Autodesk Inventor part; units mm, degrees
ref_plane "YZ Plane" through (0, 0, 0) normal (1, 0, 0) x (0, 1, 0)
ref_plane "XZ Plane" through (0, 0, 0) normal (0, 1, 0) x (-1, 0, 0)
ref_plane "XY Plane" through (0, 0, 0) normal (0, 0, 1) x (1, 0, 0)
sketch "Sketch1" plane through (0, 0, 0) normal (0, 0, 1) x (1, 0, 0)
  line L0 (0, 0) -> (3.75, 0)
  line L1 (3.75, 0) -> (3.75, -5)
  line L2 (3.75, -5) -> (11.25, -5)
  line L3 (11.25, -5) -> (11.25, 0)
  line L4 (11.25, 0) -> (21.731, 0)
  line L5 (21.731, 0) -> (21.731, 50)
  line L6 (21.731, 50) -> (11.25, 50)
  line L7 (11.25, 50) -> (11.25, 55)
  line L8 (11.25, 55) -> (3.75, 55)
  line L9 (3.75, 55) -> (3.75, 50)
  line L10 (3.75, 50) -> (0, 50)
  line L11 (0, 50) -> (0, 0)
  line L12 (21.731, 35) -> (15, 35)
  line L13 (15, 35) -> (15, 15)
  line L14 (15, 15) -> (21.731, 15)
  line L15 (21.731, 15) -> (21.731, 35)
  circle A0 centre (7.5, 35) radius 1.6
  circle A1 centre (7.5, 15) radius 1.6
  line L16 (7.5, 15) -> (7.5, 35)
  point P0 (21.731, 25)
  point P1 (21.731, 25)
  point P2 (7.5, -5)
  point P3 (7.5, 25)
  point P4 (0, 25)
  dimension "d0" = 50
  dimension "d1" = 3.75
  dimension "d2" = 5
  dimension "d3" = 7.5
  dimension "d4" = 10.481
  dimension "d5" = 6.731
  dimension "d6" = 20
  dimension "d7" = 3.75
  dimension "d10" = 3.2
  dimension "d11" = 20
extrude "Extrusion1" add sketch "Sketch1" along normal blind 6.731 contours L11 L10 L9 L8 L7 L6 L5 L12 L13 L14 L4 L3 L2 L1 L0
equation "\"d4\" = d7 + THICKB"
equation "\"d5\" = THICKB"
equation "\"d7\" = d1"
equation "\"d8\" = THICKB"
equation "\"THICKA\" = 3.175"
equation "\"THICKB\" = 6.731"
equation "\"THICKC\" = 12.7"
equation "\"BALLDIA\" = 12"
equation "\"MAGDIA\" = 9.5"
equation "\"THICKPLY\" = 5"
properties part number "Frame_Lower_Vertical_Plate_A"
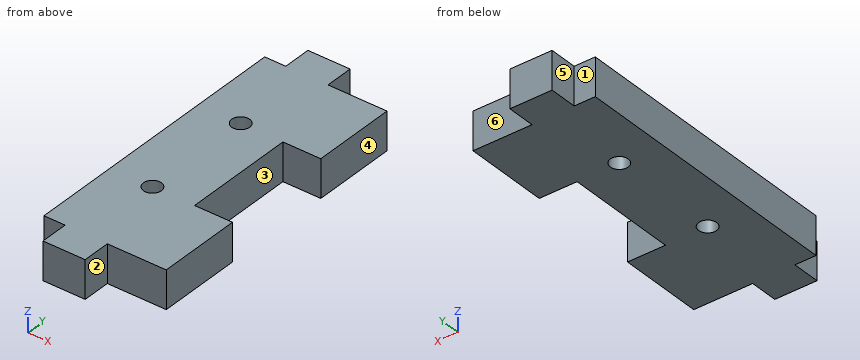
Input: part model. Units: mm. Frame: model coordinates. Face numbers are marked on the shaded views. A direction names the side the tool comes from. Give positions to 0.01 mm unless a question says otherwise; leave off trailing zeros. Loops run counter-clockwise (first coordinate to the right, second up) from the corner with the lowest first, then second, coordinate; pieces in that order, holes last. Notation, with made-up numbers: (85, -16.5) - (122, -16.5) arc R18 ccw to (122, -1.5) - close; hole circle Ø7 at (13.5, 4). An arc over 180 degrees is marked (long way). Use CSV: the item, a comma, the result in double quotes. Start each with the question number.
Item 1: Section D-D on x = 2.75. Return loops of the section in (y, z).
Item 2: Reachability of the marked faces 1, 2 and 3 from +Z, -Z, +X, -X, +Y, -Y: full face, straight path, thin tool, end or side. Return the list, or none.
Item 3: Section B-B on z = 5. Return loops of the section in (x, y).
Item 4: Section C-C on x = 16.75. Return loops of the section in (y, z), then the cut area to 3 significant figures.
Item 5: Mould query, pull axis X, two halves, no side actions, for the marked faces 4, 5 and 6. Classes: pulls with the +X half, pulls with the -X half, needs draft (parallel to the pull), parting line crosses it, or undercut.
Item 6: Line query: line 1 (Y direction, x = 7.5, z = 2.25); line 2 (Y direction, x = 19.75, z = 6.5); line 3 (Y direction, x = 2.5, z = 3.75). Output: solid intervals per line, ascending.
Item 7: Contact query for flat-ended pins moving along their axis: P1, Ø1, axis at x = 18.5, z = 4.5, coming from the -Y side; P2, Ø4, axis at x = 7.5, y = 35.5, coming from the +Z side; P3, Ø4, axis at y = -2.5, z = 4.5, coming from the +X side; P4, Ø4, axis at y = 52.5, z = 3, coming from the -X side. Output: stop coordinate, or through.
Item 8: Section A-A on x = 7.5. Return loops of the section in (y, z), then the cut area to 3 significant figures.
Ans:
1,outline,"(0, 0) - (50, 0) - (50, 6.73) - (0, 6.73) - close"
2,face 1,"+Z, -Z, -X, +Y"
2,face 2,"+Z, -Z, +X, -Y"
2,face 3,"+Z, -Z, +X"
3,outline,"(0, 0) - (3.75, 0) - (3.75, -5) - (11.25, -5) - (11.25, 0) - (21.73, 0) - (21.73, 15) - (15, 15) - (15, 35) - (21.73, 35) - (21.73, 50) - (11.25, 50) - (11.25, 55) - (3.75, 55) - (3.75, 50) - (0, 50) - close; hole circle Ø3.2 at (7.5, 15); hole circle Ø3.2 at (7.5, 35)"
4,outline,"(0, 0) - (15, 0) - (15, 6.73) - (0, 6.73) - close; (35, 0) - (50, 0) - (50, 6.73) - (35, 6.73) - close"
4,area,"202 mm2"
5,face 4,"pulls with the +X half"
5,face 5,"pulls with the -X half"
5,face 6,"needs draft"
6,line 1,"y = -5 to 13.4, 16.6 to 33.4, 36.6 to 55"
6,line 2,"y = 0 to 15, 35 to 50"
6,line 3,"y = 0 to 50"
7,P1,"stops at y = 0"
7,P2,"stops at z = 6.73"
7,P3,"stops at x = 11.25"
7,P4,"stops at x = 3.75"
8,outline,"(-5, 0) - (13.4, 0) - (13.4, 6.73) - (-5, 6.73) - close; (16.6, 0) - (33.4, 0) - (33.4, 6.73) - (16.6, 6.73) - close; (36.6, 0) - (55, 0) - (55, 6.73) - (36.6, 6.73) - close"
8,area,"361 mm2"
